CAD build for the part. Positions are in the model's coordinates, mm. Face numbers are marked on the shaded views. A direction names the side the tool comes from. Give positions to 0.01 mm unless a question says otherwise; leave off trailing zeros. Write each loop counter-clockwise with the first axis right and the second up, starting at its lowest first coordinate (ties: lowest second). Pieces come first, ordered by that corner, then holes. Notation, with made-up numbers: (69, -31.75) -> (117, -31.75) arc R4 ccw to (117, -25.75) -> close; hole circle Ø9 at (24.5, 13.25). An arc over 180 degrees is marked (long way). Answer in a Markdown table with one row per item. Add a question column.
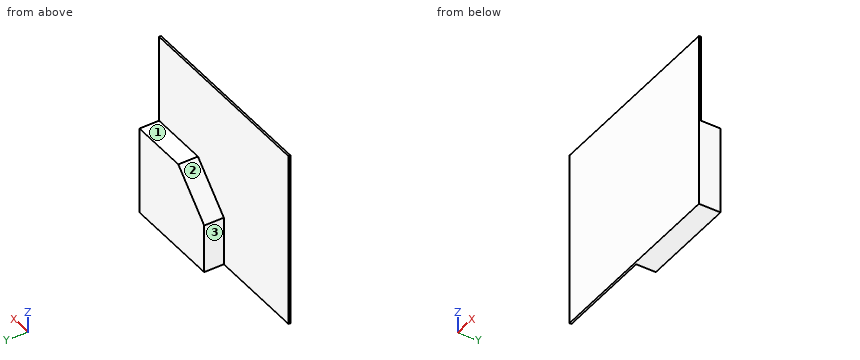
```python
from build123d import *

# Parameters (mm, degrees)
SKETCH1_W           = 1000
SKETCH1_H           = 900
BOSS_EXTRUDE1_DEPTH = 10
BOSS_EXTRUDE2_DEPTH = 100


with BuildPart() as part:
    # Sketch1 → Boss-Extrude1 (new body)
    with BuildSketch(Plane(origin=(0, 0, 0), x_dir=(1, 0, 0), z_dir=(0, 1, 0))):
        Rectangle(SKETCH1_W, SKETCH1_H)
    extrude(amount=BOSS_EXTRUDE1_DEPTH)

    # Sketch2 → Boss-Extrude2 (add)
    with BuildSketch(Plane(origin=(0, 10, 0), x_dir=(1, 0, 0), z_dir=(0, 1, 0))):
        Polygon((0, 450), (0, 200), (200, 0), (500, 0), (500, 450), align=None)
    extrude(amount=BOSS_EXTRUDE2_DEPTH)


solid = part.part
```
Item 1: Drop flat-ended pins along their axis: pin 1 Ø12 at (x, z) = (59.5, 8) entering from +Y; pin 2 Ø8 at (y, z) = (26, -248) entering from -X; pin 3 Ø1 at (x, z) = (111.5, -154.5) entering from -Y. Give the stop position or say it passes through.
Item 2: Slice it at B-B, the plane z = -375.5. List the corners of the cut face in (x, y), then the cut area to 3 significant figures.
Item 3: Probe L1, parallel to Z at x = 395.5, y = 74.5; L2, parallel to Y at x = 4, z = 265; L3, parallel to X at y = 69.5, z = -347.5. List the from-to ranges inside material, lowest first. Write a range as from..to.
Item 4: Which spindle directions (+Z, -Z, +X, -X, +Y, -Y) get a long thin tool onto all of the face, cutting with end or side? Do the marked faces 1, 2 and 3. Say none if no direction does.
Item 5: Slice it at C-C, the plane y = 44. List the corners of the cut face in (x, z).
Item 6: Slice it at A-A, the plane x = 59. List the corners of the cut face in (y, z), then the cut area to 3 significant figures.
Item 7: Slice it at D-D, the plane x = -172.5. List the corners of the cut face in (y, z), then the cut area to 3 significant figures.
Answer key:
| question | item | result |
|---|---|---|
| 1 | pin 1 | stops at y = 10 |
| 1 | pin 2 | stops at x = 0 |
| 1 | pin 3 | stops at y = 0 |
| 2 | outline | (-500, 0) -> (500, 0) -> (500, 110) -> (0, 110) -> (0, 10) -> (-500, 10) -> close |
| 2 | area | 60,000 mm² |
| 3 | L1 | z = -450..0 |
| 3 | L2 | y = 0..10 |
| 3 | L3 | x = 0..500 |
| 4 | face 1 | +Z, +X, -X, +Y |
| 4 | face 2 | +Z, -X, +Y |
| 4 | face 3 | +Z, -Z, -X, +Y |
| 5 | outline | (0, -450) -> (500, -450) -> (500, 0) -> (200, 0) -> (0, -200) -> close |
| 6 | outline | (0, -450) -> (110, -450) -> (110, -141) -> (10, -141) -> (10, 450) -> (0, 450) -> close |
| 6 | area | 39,900 mm² |
| 7 | outline | (0, -450) -> (10, -450) -> (10, 450) -> (0, 450) -> close |
| 7 | area | 9,000 mm² |
